Answer from the drawing. Dimensions are ordinates in mm from the lowest x, y and z of the part. A direction names the side the tool comes from. Coordinates: 2 decimals unless noted, no trailing zeros. Loops run counter-clockwise (first coordinate to the right, second up) from the corner with the lowest first, then second, coordinate; pieces in that order, holes last. Notation, with made-up numbers: (-32, 86) - (-23, 86) arc R34 cw to (-23, 118) - close; hole circle Ø10 at (4.5, -4). An arc over 180 degrees is marked (long way). Use one line per item in the form item = value. Start each with the question number.
1) Each of these flat-tipped pins is pushed along its axis until it touches: P1, Ø1, axis at x = 23, z = 31.5, coming from the +Y side; P2, Ø1.5, axis at x = 26, z = 44, coming from the +Y side (1 decimal); P3, Ø2, axis at x = 19.5, z = 39.5, coming from the -Y side (1 decimal). Where does it stop, or does it pass through?
2) Which of the six approach directions +Z, -Z, +X, -X, +Y, -Y give full straight-line access (tool end or side, diameter ignored) to the marked faces 1 and 2?
3) A cutting plane is placed at A-A (z = 44.5). Give the vertices of the cut face in (x, y) (1 decimal).
4) Consider line 1 (Z direction, x = 27, y = 22) (1 decimal); line 2 (Y direction, x = 22.5, z = 33); line 3 (Z direction, x = 13, y = 23). Determine where each line is inside the solid, lowest interval first.
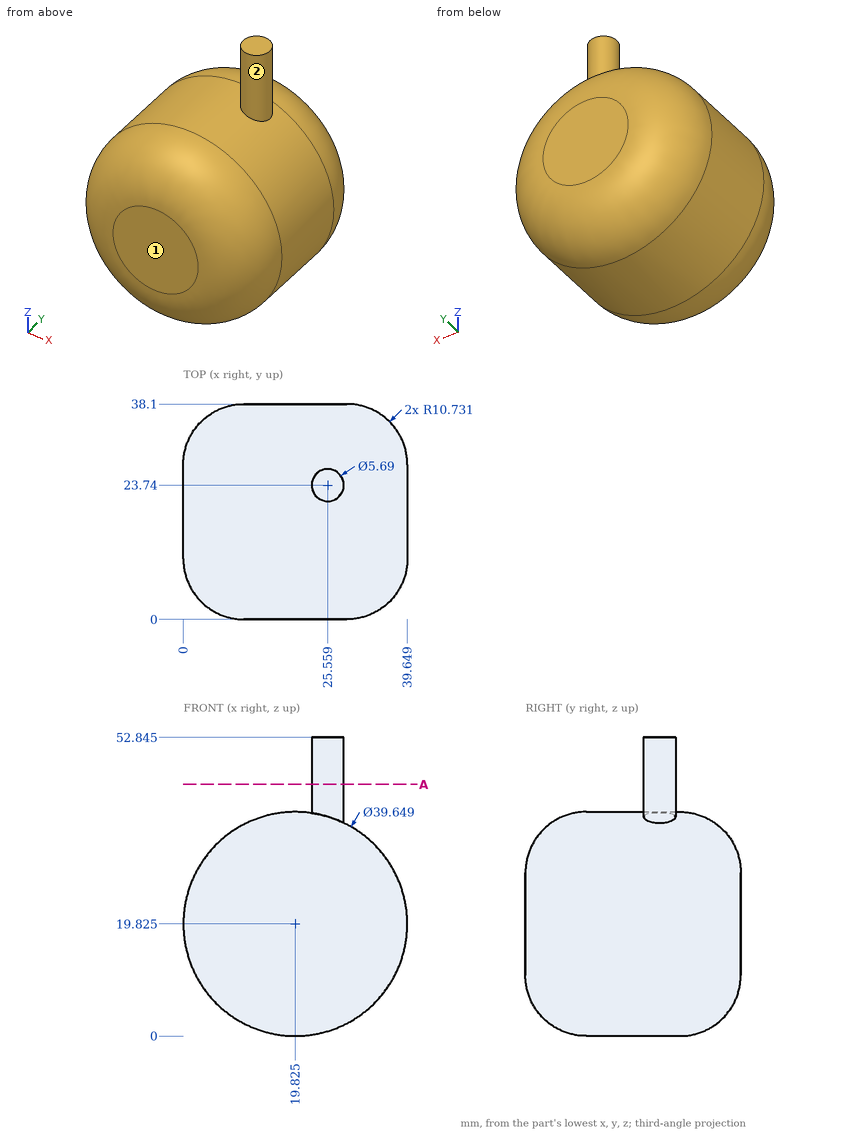
Found:
q1.P1 = 37.8
q1.P2 = 26.6
q1.P3 = 5.9
q2.face_1 = +Z, -Z, +X, -X, -Y
q2.face_2 = +Z
q3.outline = circle Ø5.7 at (25.6, 23.7)
q4.line_1 = 1.3 to 52.8
q4.line_2 = 0.92 to 37.18
q4.line_3 = 1.21 to 38.44
